Build history of the part. All positions in model axes, mm. A direction names the side the tool comes from. Round coordinates to 2 decimals unless told otherwise and drop trailing zeros. Write each loop counter-clockwise with the first axis right and the second up, starting at its lowest first coordinate (ties: lowest second). Pieces come first, ordered by that corner, then holes.
1) Saw through at B-B (z = 12.7). Write the cut outline in (x, y) (3 decimals), plus the area to 3 significant figures.
2) Flat gauge pin, fed straight in: pin 1 (5 mm diameter, centred on x = 0, z = 12.7, fed in from -Y). Where does the tip first touch, or does it go through?
3) Which spindle directions (+Z, -Z, +X, -X, +Y, -Y) get a long thin tool onto all of the face, cutting with end or side? Do faces 1 (the cylindrical face through (-1.205, 1.521, 16.528)), 2 (the flat face through (12.7, 0, 0)). Say none if no direction does.
4) Pull direction X, two halves, no side cores. Call faces 3 (the flat face through (-12.7, 0, 0)), 4 (the flat face through (3, -3.175, -15)), 5 (the flat face through (0, -6.35, 0)): +X half, -X half, draft (parallel to the pull), parting line (faces both ways), or undercut.
5) Saw through at C-C (y = -2.5). Write the cut outline in (x, z).
6) Saw through at A-A (x = 0). Write the cut outline in (y, z) (3 decimals), plus the area to 3 significant figures.
7) Saw through at D-D (z = -10.5). Write the cut outline in (x, y) (3 decimals).
8) Wall check: probe 1 along Z at (x, y) = (0, -4.1); probe 2 along Z at (x, y) = (0, 3); probe 3 along X at (y, z) = (-0.75, 12.7). Give the ranges that are in metal, low to high.
Autodesk Inventor part; units mm, degrees
ref_plane "YZ Plane" through (0, 0, 0) normal (1, 0, 0) x (0, 1, 0)
ref_plane "XZ Plane" through (0, 0, 0) normal (0, 1, 0) x (-1, 0, 0)
ref_plane "XY Plane" through (0, 0, 0) normal (0, 0, 1) x (1, 0, 0)
sketch "Sketch1" plane through (0, 0, 0) normal (0, 0, 1) x (1, 0, 0)
  line L0 (-12.7, -6.35) -> (12.7, -6.35)
  line L1 (12.7, -6.35) -> (12.7, 6.35)
  line L2 (12.7, 6.35) -> (-12.7, 6.35)
  line L3 (-12.7, 6.35) -> (-12.7, -6.35)
  line L4 (-12.7, -6.35) -> (12.7, 6.35) construction
  line L5 (12.7, -6.35) -> (-12.7, 6.35) construction
  point P0 (0, 0)
  dimension "d0" = 25.4
  dimension "d1" = 12.7
extrude "Extrusion1" add sketch "Sketch1" along normal mid plane 50.8
sketch "Sketch2" plane through (-12.7, 6.35, 25.4) normal (0, 1, 0) x (1, 0, 0)
  line L0 (25.4, 0) -> (0, 0)
  line L1 (0, 50.8) -> (25.4, 50.8)
  point P0 (12.7, 25.4)
  point P1 (12.7, 12.7)
  point P2 (12.7, 38.1)
  dimension "d11" = 12.7
  dimension "d12" = 12.7
hole "Hole1" at (0, 6.35, 12.7) at (0, 6.35, -12.7) direction (0, -1, 0) diameter 6.7564 end through all counterbore diameter 8.0264 counterbore depth 9.525
properties part number "seatingPartsExample" material "Phenolic Resin"
Evaluation:
1. outline: (-12.7, -6.35) - (-3.378, -6.35) - (-3.378, -3.175) - (-4.013, -3.175) - (-4.013, 6.35) - (-12.7, 6.35) - close; (3.378, -6.35) - (12.7, -6.35) - (12.7, 6.35) - (4.013, 6.35) - (4.013, -3.175) - (3.378, -3.175) - close
1. area: 225 mm2
2. pin 1: passes through
3. face 1: +Y
3. face 2: +Z, -Z, +X, +Y, -Y
4. face 3: -X half
4. face 4: undercut
4. face 5: draft
5. outline: (-12.7, -25.4) - (12.7, -25.4) - (12.7, 25.4) - (-12.7, 25.4) - close; hole circle Ø8.03 at (0, -12.7); hole circle Ø8.03 at (0, 12.7)
6. outline: (-6.35, -25.4) - (6.35, -25.4) - (6.35, -16.713) - (-3.175, -16.713) - (-3.175, -16.078) - (-6.35, -16.078) - close; (-6.35, -9.322) - (-3.175, -9.322) - (-3.175, -8.687) - (6.35, -8.687) - (6.35, 8.687) - (-3.175, 8.687) - (-3.175, 9.322) - (-6.35, 9.322) - close; (-6.35, 16.078) - (-3.175, 16.078) - (-3.175, 16.713) - (6.35, 16.713) - (6.35, 25.4) - (-6.35, 25.4) - close
6. area: 449 mm2
7. outline: (-12.7, -6.35) - (-2.564, -6.35) - (-2.564, -3.175) - (-3.356, -3.175) - (-3.356, 6.35) - (-12.7, 6.35) - close; (2.564, -6.35) - (12.7, -6.35) - (12.7, 6.35) - (3.356, 6.35) - (3.356, -3.175) - (2.564, -3.175) - close
8. probe 1: z = -25.4 to -16.08, -9.32 to 9.32, 16.08 to 25.4
8. probe 2: z = -25.4 to -16.71, -8.69 to 8.69, 16.71 to 25.4
8. probe 3: x = -12.7 to -4.01, 4.01 to 12.7
